Design review of the part built by this model. Coordinates are the model's own, in mm. A direction names the side the tool comes from. Give positions to 0.01 mm unless a question says otherwise; leave off trailing zeros. Write each loop counter-clockwise with the first axis right and the second up, starting at its lowest first coordinate (ties: lowest second). Pieces come first, ordered by that corner, then holes. Notation, with made-up numbers: (-8.75, 47.5) -> (33.25, 47.5) arc R25 cw to (33.25, 74.5) -> close; hole circle Ø7 at (30, 27.25). An arc over 180 degrees is marked (long way). Write each question's results on one line, items separated by ' | '. Start each with the question number.
(1) Take a section at B-B (z = 0). State the section outline as (x, y) points.
(2) Take a section at C-C (x = 0). State the section outline as (y, z) points, plus the area to 3 significant figures.
(3) Take a section at A-A (y = 10.5). State the section outline as (x, z) points.
(4) Take a section at D-D (y = 26). State the section outline as (x, z) points, plus the area to 3 significant figures.
(5) Clearance check with flat-ended pins moving along their axes: pin 1 (1.5 mm diameter, centred on x = -18.5, y = 49, fed in from +Z); pin 2 (22 mm diameter, centred on y = 26, z = -10, fed in from +X); pin 3 (10 mm diameter, centred on y = 8.5, z = -8.5, fed in from -X); pin 4 (4.5 mm diameter, centred on x = 18.01, z = -30.5, fed in from -Y). State where each tip first meets the part, or that it passes through.
(6) For faces 3 (the face through (19, 44, 0)), 4 (the face through (-23, 49, 9.5)), 5 (the face through (-31, 9, 24)), 6 (the face through (-32, 27, -23)), list the 3-axis set-ups (+Z, -Z, +X, -X, +Y, -Y) from which the entire face can be reached by the end or side of a thin tool; tool diameter is ignored.
(7) To check wall thickness, follow probe 1 along X at (y, z) = (3, 0); probe 2 along Y at (x, z) = (11, -3.5); probe 3 along Z at (x, y) = (7, 21). State the ranges of each line that lie inside material, in increasing order.
(8) Mouldability with a two-part tool opening along Y and no side actions: class faces 1 (the face through (10, 26, -22)), 2 (the face through (20, 27, -13)) as released by +Y, released by -Y, zero draft, split by the parting line, or undercut.
from build123d import *

# Parameters (mm, degrees)
SKETCH_1_R          = 40
SKETCH_1_R_2        = 2
EXTRUDE_1_DEPTH     = 4
EXTRUDE_2_DEPTH     = 44
EXTRUDE_4_DEPTH     = 3
SKETCH_5_R          = 1.5
SKETCH_5_R_2        = 11.25
CUT_EXTRUDE_1_DEPTH = 87.313382508
SKETCH_6_W          = 6
SKETCH_6_H          = 25
CUT_EXTRUDE_2_DEPTH = 3
SKETCH_8_R          = 2
CUT_EXTRUDE_3_DEPTH = 74.545904097
SKETCH_9_R          = 4
CUT_EXTRUDE_4_DEPTH = 3


with BuildPart() as part:
    # 草图1 → 凸台-拉伸1 (new body)
    with BuildSketch(Plane(origin=(0, 0, 0), x_dir=(1, 0, 0), z_dir=(0, 1, 0))):
        with Locations(Location((0, 0, 0), (0, 0, 270))):
            Circle(SKETCH_1_R)
        with Locations(Location((0, 23, 0), (0, 0, 270))):
            Circle(SKETCH_1_R_2, mode=Mode.SUBTRACT)
        with Locations(Location((23, 0, 0), (0, 0, 270))):
            Circle(SKETCH_1_R_2, mode=Mode.SUBTRACT)
        with Locations(Location((0, -23, 0), (0, 0, 270))):
            Circle(SKETCH_1_R_2, mode=Mode.SUBTRACT)
        with Locations(Location((-23, 0, 0), (0, 0, 270))):
            Circle(SKETCH_1_R_2, mode=Mode.SUBTRACT)
    extrude(amount=EXTRUDE_1_DEPTH)

    # 草图2 → 凸台-拉伸2 (add)
    with BuildSketch(Plane(origin=(0, 4, 0), x_dir=(1, 0, 0), z_dir=(0, 1, 0))):
        with BuildLine():
            Line((-33, 22), (-3.872983346, 22))
            ThreePointArc((-3.872983346, 22), (-3.963357659, 23.540181513), (-3.464101615, 25))
            Line((-3.464101615, 25), (-30, 25))
            Line((-30, 25), (-33, 22))
        make_face()
        with BuildLine():
            Line((-33, -22), (-3.872983346, -22))
            ThreePointArc((-3.872983346, -22), (-3.963357659, -23.540181513), (-3.464101615, -25))
            Line((-3.464101615, -25), (-30, -25))
            Line((-30, -25), (-33, -22))
        make_face()
        with BuildLine():
            Line((17, 22), (17, -22))
            Line((17, -22), (3.872983346, -22))
            ThreePointArc((3.872983346, -22), (3.963357659, -23.540181513), (3.464101615, -25))
            Line((3.464101615, -25), (17.525126266, -25))
            Line((17.525126266, -25), (20, -22.525126266))
            Line((20, -22.525126266), (20, -2.645751311))
            ThreePointArc((20, -2.645751311), (19, 0), (20, 2.645751311))
            Line((20, 2.645751311), (20, 22.525126266))
            Line((20, 22.525126266), (17.525126266, 25))
            Line((17.525126266, 25), (3.464101615, 25))
            ThreePointArc((3.464101615, 25), (3.963357659, 23.540181513), (3.872983346, 22))
            Line((3.872983346, 22), (17, 22))
        make_face()
    extrude(amount=EXTRUDE_2_DEPTH)

    # 草图3 → 凸台-拉伸4 (add)
    with BuildSketch(Plane(origin=(0, 48, 0), x_dir=(1, 0, 0), z_dir=(0, 1, 0))):
        with BuildLine():
            Line((-3.464101615, 25), (3.464101615, 25))
            Line((3.464101615, 25), (17.525126266, 25))
            Line((17.525126266, 25), (20, 22.525126266))
            Line((20, 22.525126266), (20, 2.645751311))
            ThreePointArc((20, 2.645751311), (19, 0), (20, -2.645751311))
            Line((20, -2.645751311), (20, -22.525126266))
            Line((20, -22.525126266), (17.525126266, -25))
            Line((17.525126266, -25), (3.464101615, -25))
            Line((3.464101615, -25), (-3.464101615, -25))
            Line((-3.464101615, -25), (-30, -25))
            Line((-30, -25), (-33, -22))
            Line((-33, -22), (-33, -9.5))
            Line((-33, -9.5), (-23, -9.5))
            Line((-23, -9.5), (-13, -9.5))
            Line((-13, -9.5), (-13, -7.5))
            Line((-13, -7.5), (-13, 7.5))
            Line((-13, 7.5), (-13, 9.5))
            Line((-13, 9.5), (-23, 9.5))
            Line((-23, 9.5), (-33, 9.5))
            Line((-33, 9.5), (-33, 22))
            Line((-33, 22), (-30, 25))
            Line((-30, 25), (-3.464101615, 25))
        make_face()
    extrude(amount=EXTRUDE_4_DEPTH)

    # 草图5 → 切除-拉伸1 (cut, through all)
    with BuildSketch(Plane.ZY.offset(-17)):
        with Locations((15.5, 41.5)):
            Circle(SKETCH_5_R)
        with Locations((-15.5, 41.5)):
            Circle(SKETCH_5_R)
        with Locations((-15.5, 10.5)):
            Circle(SKETCH_5_R)
        with Locations((15.5, 10.5)):
            Circle(SKETCH_5_R)
        with Locations((0, 26)):
            Circle(SKETCH_5_R_2)
    extrude(amount=-CUT_EXTRUDE_1_DEPTH, mode=Mode.SUBTRACT)

    # 草图6 → 切除-拉伸2 (cut)
    with BuildSketch(Plane.XY.offset(25)):
        with Locations((-30, 26)):
            Rectangle(SKETCH_6_W, SKETCH_6_H)
    extrude(amount=-CUT_EXTRUDE_2_DEPTH, mode=Mode.SUBTRACT)

    # 草图8 → 切除-拉伸3 (cut, through all)
    with BuildSketch(Plane(origin=(0, 4, 0), x_dir=(1, 0, 0), z_dir=(0, 1, 0))):
        with Locations(Location((18.014281267, 30.496919032, 0), (0, 0, 270))):
            Circle(SKETCH_8_R)
        with Locations(Location((18.014281267, -30.496919032, 0), (0, 0, 90))):
            Circle(SKETCH_8_R)
        with Locations(Location((-18.014281267, -30.496919032, 0), (0, 0, 270))):
            Circle(SKETCH_8_R)
        with Locations(Location((-18.014281267, 30.496919032, 0), (0, 0, 90))):
            Circle(SKETCH_8_R)
    extrude(amount=-CUT_EXTRUDE_3_DEPTH, mode=Mode.SUBTRACT)

    # 草图9 → 切除-拉伸4 (cut)
    with BuildSketch(Plane(origin=(0, 4, 0), x_dir=(1, 0, 0), z_dir=(0, 1, 0))):
        with Locations(Location((-23, 0, 0), (0, 0, 270))):
            Circle(SKETCH_9_R)
    extrude(amount=-CUT_EXTRUDE_4_DEPTH, mode=Mode.SUBTRACT)


solid = part.part
Report:
1) outline: (-40, 0) -> (-25, 0) -> (-25, 1) -> (-27, 1) -> (-27, 4) -> (-40, 4) -> close; (-21, 0) -> (21, 0) -> (21, 4) -> (19, 4) -> (19, 14.75) -> (17, 14.75) -> (17, 4) -> (-19, 4) -> (-19, 1) -> (-21, 1) -> close; (-13, 48) -> (17, 48) -> (17, 37.25) -> (19, 37.25) -> (19, 51) -> (-13, 51) -> close; (25, 0) -> (40, 0) -> (40, 4) -> (25, 4) -> close
2) outline: (0, -40) -> (4, -40) -> (4, -25) -> (0, -25) -> close; (0, -21) -> (4, -21) -> (4, 21) -> (0, 21) -> close; (0, 25) -> (4, 25) -> (4, 40) -> (0, 40) -> close; (48, -25) -> (51, -25) -> (51, 25) -> (48, 25) -> close | area: 438 mm2
3) outline: (-33, -22) -> (-30, -25) -> (-3.46, -25) arc R4 cw to (-3.87, -22) -> close; (-33, 22) -> (-3.87, 22) arc R4 cw to (-3.46, 25) -> (-30, 25) -> close; (3.46, -25) -> (17.53, -25) -> (20, -22.53) -> (20, -17) -> (17, -17) -> (17, -22) -> (3.87, -22) arc R4 cw to start; (3.46, 25) arc R4 cw to (3.87, 22) -> (17, 22) -> (17, 17) -> (20, 17) -> (20, 22.53) -> (17.53, 25) -> close; (17, -14) -> (20, -14) -> (20, -2.65) arc R4 cw to (20, 2.65) -> (20, 14) -> (17, 14) -> close
4) outline: (-33, -22) -> (-30, -25) -> (-3.46, -25) arc R4 cw to (-3.87, -22) -> close; (-27, 22) -> (-3.87, 22) arc R4 cw to (-3.46, 25) -> (-27, 25) -> close; (3.46, -25) -> (17.53, -25) -> (20, -22.53) -> (20, -11.25) -> (17, -11.25) -> (17, -22) -> (3.87, -22) arc R4 cw to start; (3.46, 25) arc R4 cw to (3.87, 22) -> (17, 22) -> (17, 11.25) -> (20, 11.25) -> (20, 22.53) -> (17.53, 25) -> close | area: 307 mm2
5) pin 1: z = 25 | pin 2: x = 20 | pin 3: x = -39.5 | pin 4: y = 0
6) face 3: +X, +Y | face 4: -X, +Y | face 5: +Z, -X, +Y | face 6: -Z, -X, +Y
7) probe 1: -40 to -27, -19 to 21, 25 to 40 | probe 2: 0 to 4, 48 to 51 | probe 3: -25 to -22, 22 to 25
8) face 1: undercut | face 2: zero draft
